Input: part model. Units: mm. Frame: model coordinates. Face numbers are marked on the shaded views. A direction names the side the tool comes from. Round coordinates to 2 decimals unless told otherwise and drop trailing zeros. Loops run counter-clockwise (first coordinate to the right, second up) from the corner with the lowest first, then second, coordinate; pieces in that order, holes last. Notation, with made-up numbers: (70.5, 5.5) - (123.5, 5.5) arc R27 ccw to (123.5, 36.5) - close; hole circle Ø8 at (-21, 40). An arc over 180 degrees is marked (long way). Use CSV: the item, a comma, the result in double quotes. Start each with the question number.
1. Pin query (flat end, axial travel): P1, Ø3, axis at y = 7.5, z = 12, coming from the +X side; P2, Ø3, axis at y = 5.5, z = 7, coming from the -X side; P3, Ø2.5, axis at x = 0, y = -6, coming from the -Z side; P4, Ø8, axis at y = -2.5, z = 3, coming from the -X side. Return the tip coordinate at first contact, or that it passes through.
2. Material intervals for probe 1 along Z at (x, y) = (2, 2.75); probe 2 along X at (y, z) = (6, 1.7), sorted ascending. Write a range as from..to.
3. Cut plane B-B (z = 1). Return loops of the section in (x, y).
4. Cut plane D-D (z = 17.25). Return loops of the section in (x, y), and give its area (3 significant figures).
5. Access query for the marked faces 1, 2 and 3. Directions: +Z, -Z, +X, -X, +Y, -Y. A direction counts if a zero-diameter tool reaches every point of the face in a straight line with its end or side. Return the directions, or none.
6. Cut plane A-A (y = 0). Return loops of the section in (x, z), and give its area (3 significant figures).
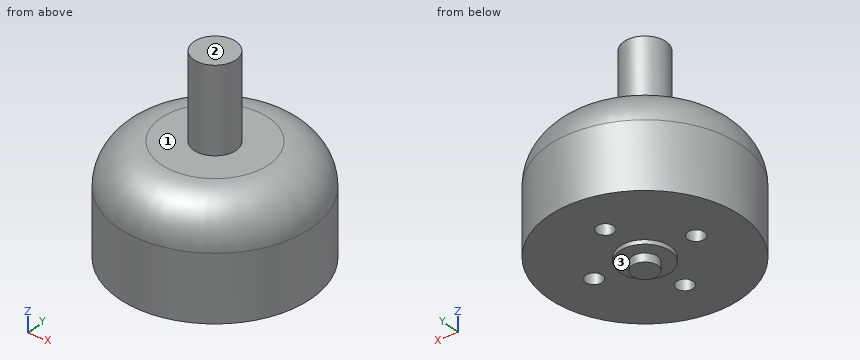
```python
from build123d import *

# Parameters (mm, degrees)
SKETCH_1_R               = 11.4
EXTRUDE_1_DEPTH          = 12.8
SKETCH_2_R               = 1
CUT_EXTRUDE_1_DEPTH      = 3
PATTERN_CIRCULAR_1_COUNT = 4
SKETCH_3_R               = 3
EXTRUDE_2_DEPTH          = 0.5
SKETCH_4_R               = 1.5
EXTRUDE_3_DEPTH          = 1
SKETCH_5_R               = 2.5
EXTRUDE_4_DEPTH          = 10
FILLET_1_R               = 5


with BuildPart() as part:
    # Sketch 1 → Extrude 1 (new body)
    with BuildSketch(Plane.XY):
        Circle(SKETCH_1_R)
    extrude(amount=EXTRUDE_1_DEPTH)

    # Sketch 2 → Cut-Extrude 1 (cut)
    with BuildSketch(Plane(origin=(0, 0, 0), x_dir=(-1, 0, 0), z_dir=(0, 0, -1))):
        with Locations((6, 0)):
            Circle(SKETCH_2_R)
    cut_extrude_1 = extrude(amount=-CUT_EXTRUDE_1_DEPTH, mode=Mode.SUBTRACT)

    # Pattern Circular 1: Cut-Extrude 1 ×4 about axis
    pattern_circular_1_axis = Axis((0, 0, 0), (0, 0, 1))
    for i in range(1, PATTERN_CIRCULAR_1_COUNT):
        add(cut_extrude_1.rotate(pattern_circular_1_axis, i * 360 / PATTERN_CIRCULAR_1_COUNT), mode=Mode.SUBTRACT)

    # Sketch 3 → Extrude 2 (add)
    with BuildSketch(Plane(origin=(0, 0, 0), x_dir=(-1, 0, 0), z_dir=(0, 0, -1))):
        Circle(SKETCH_3_R)
    extrude(amount=EXTRUDE_2_DEPTH)

    # Sketch 4 → Extrude 3 (add)
    with BuildSketch(Plane(origin=(0, 0, -0.5), x_dir=(-1, 0, 0), z_dir=(0, 0, -1))):
        Circle(SKETCH_4_R)
    extrude(amount=EXTRUDE_3_DEPTH)

    # Sketch 5 → Extrude 4 (add)
    with BuildSketch(Plane.XY.offset(12.8)):
        Circle(SKETCH_5_R)
    extrude(amount=EXTRUDE_4_DEPTH)

    # Fillet 1
    fillet_1_edges = [part.edges().sort_by_distance(p)[0] for p in [
        (-11.4, 0, 12.8),
    ]]
    fillet(fillet_1_edges, radius=FILLET_1_R)


solid = part.part
```
Established:
1,P1,"stops at x = 8.04"
1,P2,"stops at x = -10.68"
1,P3,"stops at z = 0"
1,P4,"stops at x = -11.4"
2,probe 1,"z = 0..12.8"
2,probe 2,"x = -9.69..-1, 1..9.69"
3,outline,"circle Ø22.8 at (0, 0); hole circle Ø2 at (-6, 0); hole circle Ø2 at (0, -6); hole circle Ø2 at (0, 6); hole circle Ø2 at (6, 0)"
4,outline,"circle Ø5 at (0, 0)"
4,area,"19.6 mm2"
5,face 1,"+Z"
5,face 2,"+Z, +X, -X, +Y, -Y"
5,face 3,"-Z"
6,outline,"(-11.4, 0) - (-7, 0) - (-7, 3) - (-5, 3) - (-5, 0) - (-3, 0) - (-3, -0.5) - (-1.5, -0.5) - (-1.5, -1.5) - (1.5, -1.5) - (1.5, -0.5) - (3, -0.5) - (3, 0) - (5, 0) - (5, 3) - (7, 3) - (7, 0) - (11.4, 0) - (11.4, 7.8) arc R5 ccw to (6.4, 12.8) - (2.5, 12.8) - (2.5, 22.8) - (-2.5, 22.8) - (-2.5, 12.8) - (-6.4, 12.8) arc R5 ccw to (-11.4, 7.8) - close"
6,area,"325 mm2"
